Design review of the part built by this model. Coordinates are the model's own, in mm. A direction names the side the tool comes from. Coordinates: 2 decimals unless noted, no trailing zeros. Loops run counter-clockwise (first coordinate to the right, second up) from the corner with the lowest first, then second, coordinate; pieces in that order, holes last. Notation, with made-up numbers: (19.25, 38.5) -> (67.25, 38.5) arc R19 cw to (67.25, 74.5) -> close; hole circle Ø5 at (52, -6.5). An arc over 180 degrees is marked (long way). One line per item, written item: value. Start each with the question number.
1. Insertion check: pin 1 (3 mm diameter, centred on x = -1, z = 0, fed in from +Y); pin 2 (1.5 mm diameter, centred on y = 1, z = 8.5, fed in from +X). Each pin has a flat end and moves straight along its axis. Give the tip position at first contact, or say it passes through.
2. Add section A-A on z = -6.5. Write out the cut boundary in (x, y).
3. For probe 1 along X at (y, z) = (0.15, 12); probe 2 along Z at (x, y) = (-1.5, 1.75); probe 3 along Z at (x, y) = (2.6, 0.2), list the stretches that pass through material, from the lowest coordinate up.
4. Machinability: for faces 4 (the flat face through (0, 0, -40.35)), 5 (the flat face through (-2, 2, 33.35)), 6 (the cylindrical face through (0.1, -2.5, -38.1)), which of the approach directions +Z, -Z, +X, -X, +Y, -Y give a long, thin tool a straight path to every point of the face, cutting with its end or side? Answer none if there is none.
5. Draft analysis for pull direction Z (two halves, no side actions). For faces 1 (the flat face through (0, 2, -36)), 2 (the conical face through (0.09, -2.64, -36.21)), 3 (the cylindrical face through (0, 2, 0)), state which applies: pulls with the +Z half, pulls with the -Z half, needs draft (parallel to the pull), parting line crosses it, or undercut.
```python
from build123d import *

# Parameters (mm, degrees)
SKETCH_1_R          = 2
EXTRUDE_1_DEPTH     = 32.35
SKETCH_2_R          = 3
EXTRUDE_2_DEPTH     = 1
SKETCH_3_R          = 2.5
EXTRUDE_3_DEPTH     = 4
EXTRUDE_START       = 4
SKETCH_4_R          = 3
EXTRUDE_4_DEPTH     = 4
SKETCH_5_R          = 2.5
EXTRUDE_5_DEPTH     = 4
CHAMFER_1_SIZE      = 0.5
CHAMFER_2_SIZE      = 0.5
SKETCH_6_W          = 6
SKETCH_6_H          = 3
CUT_EXTRUDE_6_DEPTH = 7.5
CHAMFER1_SIZE       = 1


with BuildPart() as part:
    # 草图1 → 拉伸1 (new, symmetric)
    with BuildSketch(Plane.XY):
        with Locations(Location((0, 0, 0), (0, 0, 180))):
            Circle(SKETCH_1_R)
    extrude(amount=EXTRUDE_1_DEPTH, both=True)

    # 草图2 → 拉伸2 (add)
    with BuildSketch(Plane.XY.offset(32.35)):
        Circle(SKETCH_2_R)
    extrude(amount=EXTRUDE_2_DEPTH)

    # 草图3 → 拉伸3 (add)
    with BuildSketch(Plane.XY.offset(33.35)):
        Circle(SKETCH_3_R)
    extrude(amount=EXTRUDE_3_DEPTH)

    # 草图4 → 拉伸4 (add)
    with BuildSketch(Plane(origin=(0, 0, -32.35), x_dir=(-1, 0, 0), z_dir=(0, 0, -1)).offset(EXTRUDE_START)):
        with Locations(Location((0, 0, 0), (0, 0, 180))):
            Circle(SKETCH_4_R)
    extrude(amount=-EXTRUDE_4_DEPTH)

    # 草图5 → 拉伸5 (add)
    with BuildSketch(Plane(origin=(0, 0, -36.35), x_dir=(-1, 0, 0), z_dir=(0, 0, -1)).offset(EXTRUDE_START)):
        with Locations(Location((0, 0, 0), (0, 0, 180))):
            Circle(SKETCH_5_R)
    extrude(amount=-EXTRUDE_5_DEPTH)

    # 倒角1
    chamfer_1_edges = [part.edges().sort_by_distance(p)[0] for p in [
        (-2.5, 0, 37.35),
        (-2.5, 0, -40.35),
    ]]
    chamfer(chamfer_1_edges, length=CHAMFER_1_SIZE)

    # 倒角2
    chamfer_2_edges = [part.edges().sort_by_distance(p)[0] for p in [
        (-3, 0, -36.35),
    ]]
    chamfer(chamfer_2_edges, length=CHAMFER_2_SIZE - 0.0001)  # a hair under: the kernel refuses the full size

    # 草图6 → 拉伸6 (cut)
    with BuildSketch(Plane(origin=(0, 0, -40.35), x_dir=(-1, 0, 0), z_dir=(0, 0, -1))):
        with Locations((0, 3.5)):
            Rectangle(SKETCH_6_W, SKETCH_6_H)
    extrude(amount=-CUT_EXTRUDE_6_DEPTH, mode=Mode.SUBTRACT)

    # Chamfer1
    chamfer1_edges = [part.edges().sort_by_distance(p)[0] for p in [
        (2, 0, -32.35),
        (2, 0, 32.35),
    ]]
    chamfer(chamfer1_edges, length=CHAMFER1_SIZE - 0.0001)  # a hair under: the kernel refuses the full size


solid = part.part
```
Worked answers:
1. pin 1: stops at y = 2
1. pin 2: stops at x = 1.98
2. outline: circle Ø4 at (0, 0)
3. probe 1: x = -1.99 to 1.99
3. probe 2: z = -40.05 to -31.65, 31.65 to 37.05
3. probe 3: z = -36.24 to -31.96, 31.96 to 33.35
4. face 4: -Z, +X, -X, +Y, -Y
4. face 5: +Z
4. face 6: -Z
5. face 1: needs draft
5. face 2: pulls with the -Z half
5. face 3: undercut
